Could you check a few things on this model? Use its own coordinates, in mm. A direction names the side the tool comes from. Round coordinates to 2 decimals unless told otherwise and drop trailing zeros. Loops run counter-clockwise (first coordinate to the right, second up) from the corner with the lowest first, then second, coordinate; pieces in that order, holes last. Notation, with made-up numbers: (60.25, 54) -> (81.25, 54) arc R17 cw to (81.25, 78) -> close; hole circle Ø11 at (-33.75, 33.5). An arc over 180 degrees is marked (long way). One line per item, written item: value.
Autodesk Inventor part; units mm, degrees
ref_plane "Start Plane" through (0, 0, 0) normal (0, 0, 1) x (1, 0, 0)
ref_plane "End Plane" through (0, 0, 2060) normal (0, 0, 1) x (1, 0, 0)
ref_plane "YZ Plane" through (0, 0, 0) normal (1, 0, 0) x (0, 1, 0)
ref_plane "Start Plane" through (0, 0, 0) normal (0, 0, 1) x (1, 0, 0)
ref_plane "End Plane" through (0, 0, 2060) normal (0, 0, 1) x (1, 0, 0)
sketch "Sketch" plane through (0, 0, 0) normal (0, 0, 1) x (1, 0, 0)
  line L0 (-102.997, -100.076) -> (-102.997, -90.551)
  line L1 (-102.997, -90.551) -> (-14.9225, -90.551)
  line L2 (-4.7625, -80.391) -> (-4.7625, 0)
  line L3 (-4.7625, 0) -> (0, 0) construction
  line L4 (0, 0) -> (0, -100.076) construction
  line L5 (0, -100.076) -> (-102.997, -100.076)
  line L6 (-60, 0) -> (80, 0) construction
  line L7 (0, -60) -> (0, 80) construction
  line L8 (102.997, -100.076) -> (102.997, -90.551)
  line L9 (102.997, -90.551) -> (14.9225, -90.551)
  line L10 (4.7625, -80.391) -> (4.7625, 0)
  line L11 (4.7625, 0) -> (0, 0) construction
  line L12 (0, -100.076) -> (102.997, -100.076)
  line L13 (-102.997, 100.076) -> (-102.997, 90.551)
  line L14 (-102.997, 90.551) -> (-14.9225, 90.551)
  line L15 (-4.7625, 80.391) -> (-4.7625, 0)
  line L16 (0, 100.076) -> (-102.997, 100.076)
  line L17 (102.997, 100.076) -> (102.997, 90.551)
  line L18 (102.997, 90.551) -> (14.9225, 90.551)
  line L19 (0, 100.076) -> (102.997, 100.076)
  line L20 (4.7625, 80.391) -> (4.7625, 0)
  arc A0 (-4.7625, 80.391) -> (-14.9225, 90.551) centre (-14.9225, 80.391) ccw
  arc A1 (14.9225, 90.551) -> (4.7625, 80.391) centre (14.9225, 80.391) ccw
  arc A2 (4.7625, -80.391) -> (14.9225, -90.551) centre (14.9225, -80.391) ccw
  arc A3 (-14.9225, -90.551) -> (-4.7625, -80.391) centre (-14.9225, -80.391) ccw
  line L21 (0, 140.1064) -> (0, -140.1064) construction
  line L22 (-144.1958, 0) -> (144.1958, 0) construction
  point P0 (-4.7625, -90.551)
  point P1 (4.7625, -90.551)
  point P2 (-4.7625, 90.551)
  point P3 (4.7625, 90.551)
  dimension "d1" = 100.076
  dimension "d2" = 9.525
  dimension "d3" = 102.997
  dimension "d4" = 4.7625
  dimension "d13" = 10.16
extrude "Body" add sketch "Sketch" along normal up to surface (2060 mm away) from surface at 0
sketch "Sketch4" plane through (0, 0, 0) normal (0, 0, 1) x (1, 0, 0)
  line L0 (0, 0) -> (10, 0)
ref_plane "Work Plane3" through (0, 0, 0) normal (0, -1, 0) x (1, 0, 0)
sketch "Sketch5" plane through (0, 0, 0) normal (0, -1, 0) x (1, 0, 0)
  line L0 (-2, 0) -> (12, 0)
  line L1 (-2, 2060) -> (12, 2060)
  dimension "d15" = 2060
equation "\"d1\" = 0.5 * G_H"
equation "\"d2\" = G_T1"
equation "\"d3\" = 0.5 * G_W"
equation "\"d4\" = 0.5 * G_T"
equation "\"d13\" = G_IR"
equation "\"d5\" = G_L"
equation "\"G_W\" = 205.994"
equation "\"G_H\" = 200.152"
equation "\"G_T\" = 9.525"
equation "\"G_T1\" = 9.525"
equation "\"G_IR\" = 10.16"
equation "\"G_L\" = d15"
equation "\"G_OFFSET_START\" = 0"
equation "\"G_OFFSET_END\" = 0"
equation "\"d12\" = G_OFFSET_END + B_L"
equation "\"B_L\" = 2060"
properties part number "ASTM A6/A6M - UP8 x 30 (7.88x8.11) - 81.102" material "Steel, Mild"
(1) If I drill on L1, parallel to Y at x = -29.5, z = 135; L2, parallel to X at y = -25.5, z = 1270; L3, parallel to X at y = 84.5, z = 1546, over which ranges is the centre line in solid material (lowest first)?
Recorded:
L1: -100.08 to -90.55, 90.55 to 100.08
L2: -4.76 to 4.76
L3: -5.63 to 5.63
(2) If we section it at B-B, the plane z = 601: Please give me the cut outline in (x, y), then the cut area to 3 significant figures.
Recorded:
outline: (-103, -100.08) -> (103, -100.08) -> (103, -90.55) -> (14.92, -90.55) arc R10.16 cw to (4.76, -80.39) -> (4.76, 80.39) arc R10.16 cw to (14.92, 90.55) -> (103, 90.55) -> (103, 100.08) -> (-103, 100.08) -> (-103, 90.55) -> (-14.92, 90.55) arc R10.16 cw to (-4.76, 80.39) -> (-4.76, -80.39) arc R10.16 cw to (-14.92, -90.55) -> (-103, -90.55) -> close
area: 5,740 mm²
(3) For faces 1 (the face through (0, 0, 2060)), 2 (the face through (-60, 90.551, 1016)), 3 (the face through (60, 90.551, 1016)), which set-ups out of +Z, -Z, +X, -X, +Y, -Y let a thin tool reach every point of the face, with its end or its side?
Recorded:
face 1: +Z, +X, -X, +Y, -Y
face 2: +Z, -Z, -X
face 3: +Z, -Z, +X
(4) Thinking about a two-plate mould opening in Y: for faces 4 (the face through (0, 0, 0)), 5 (the face through (1, -100.076, 1016)), 6 (the face through (4.762, 1, 1016)), which applies, released by +Y, released by -Y, zero draft, split by the parting line, or undercut?
Recorded:
face 4: zero draft
face 5: released by -Y
face 6: undercut
(5) I'm going to push flat-ended pins straight in: pin 1 Ø8 at (y, z) = (-40.5, 1551.5) entering from +X; pin 2 Ø1 at (y, z) = (-20, 865) entering from -X. Where does each tip first touch, or does it pass through?
Recorded:
pin 1: x = 4.76
pin 2: x = -4.76
(6) If we section it at C-C, the plane y = 54.5: Please give me the cut outline in (x, z), then the cut area to 3 significant figures.
Recorded:
outline: (-4.76, 0) -> (4.76, 0) -> (4.76, 2060) -> (-4.76, 2060) -> close
area: 19,600 mm²
(7) If we section it at A-A, the plane x = 46: Please give me the cut outline in (y, z), then the cut area to 3 significant figures.
Recorded:
outline: (-100.08, 0) -> (-90.55, 0) -> (-90.55, 2060) -> (-100.08, 2060) -> close; (90.55, 0) -> (100.08, 0) -> (100.08, 2060) -> (90.55, 2060) -> close
area: 39,200 mm²
